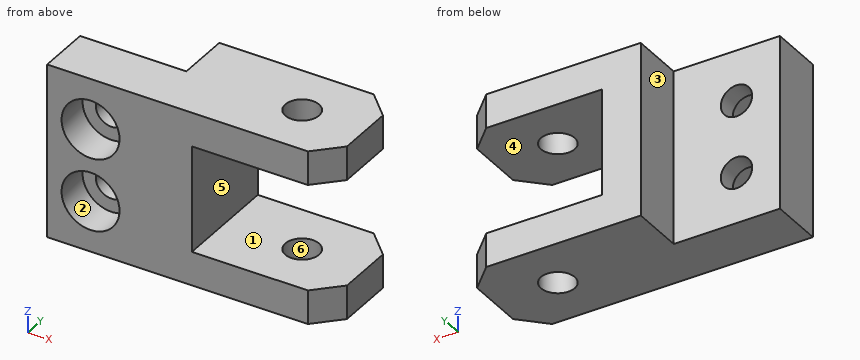
```python
from build123d import *

# Parameters (mm, degrees)
ESQUISSE1_R                                     = 3.5
BASE_EXTRUSION_DEPTH                            = 36
CHAMBRAGE_POUR_VIS_T_TE_CYLINDRIQUE_D           = 6.5
CHAMBRAGE_POUR_VIS_T_TE_CYLINDRIQUE_CBORE_D     = 12
CHAMBRAGE_POUR_VIS_T_TE_CYLINDRIQUE_CBORE_DEPTH = 7
ENL_V_MAT_EXTRU_1_DEPTH                         = 29


with BuildPart() as part:
    # Esquisse1 → Base-Extrusion (new body)
    with BuildSketch(Plane.XY):
        Polygon((0, 0), (0, 11), (32, 11), (37, 6), (37, -6), (32, -11), (-22, -11), (-22, 0), align=None)
        with Locations((24, 0)):
            Circle(ESQUISSE1_R, mode=Mode.SUBTRACT)
    extrude(amount=-BASE_EXTRUSION_DEPTH)

    # Chambrage pour vis à tête cylindrique à 6 pans creux (vis CHC) M51 (through all)
    with Locations(Plane.XZ.offset(11)):
        with Locations((-13, -25.5), (-13, -10.5)):
            CounterBoreHole(CHAMBRAGE_POUR_VIS_T_TE_CYLINDRIQUE_D / 2, CHAMBRAGE_POUR_VIS_T_TE_CYLINDRIQUE_CBORE_D / 2, CHAMBRAGE_POUR_VIS_T_TE_CYLINDRIQUE_CBORE_DEPTH)

    # Esquisse4 → Enlèv. mat.-Extru.1 (cut)
    with BuildSketch(Plane(origin=(37, 0, 0), x_dir=(0, 0, -1), z_dir=(1, 0, 0))):
        Polygon((29, -12.973294334), (18, -12.973294334), (7, -12.973294334), (7, 12.026705666), (18, 12.026705666), (29, 12.026705666), align=None)
    extrude(amount=-ENL_V_MAT_EXTRU_1_DEPTH, mode=Mode.SUBTRACT)


solid = part.part
```
CAD build for the part. Positions are in the model's coordinates, mm. Face numbers are marked on the shaded views. A direction names the side the tool comes from. Round coordinates to 2 decimals unless told otherwise and drop trailing zeros. Order: outer loops, then holes, each group sorted by start corner. A loop starts at its lowest first (then second) coordinate and runs counter-clockwise, first axis right, second up. Notation, with made-up numbers: (31, 63.5) - (71, 63.5) arc R18 cw to (71, 76.5) - close; hole circle Ø11 at (65, -3.75). An arc over 180 degrees is marked (long way). Use CSV: the item, a comma, the result in double quotes. Start each with the question number.
1) Two-plate mould, pull along X, no slides. Class the marked faces 4, 5 and 6: pulls with the +X half, pulls with the -X half, needs draft (parallel to the pull), parting line crosses it, or undercut.
2) Wall check: L1, parallel to Z at x = -13, y = -7.25; L2, parallel to Z at x = 10, y = -10; L3, parallel to Z at x = -13, y = -2.85. Give the ranges that are in metal, low to high. Write a range as [from, to].
3) Tool access for the marked faces 1, 2 and 3: list every direction of +Z, -Z, +X, -X, +Y, -Y with a clear straight run to the whole face (end or side of a thin tool).
4) Pin check, flat tips, straight feed: pin 1 Ø6 at (x, y) = (19.5, 5) entering from +Z; pin 2 Ø8.5 at (x, z) = (-13, -10.5) entering from +Y; pin 3 Ø6 at (y, z) = (7.5, -24) entering from -X; pin 4 Ø11 at (y, z) = (0.5, -13) entering from +X. Stop position of each tip, or through.
5) Saw through at D-D (y = 2.75). List the corners of the cut face in (x, z), and give its area (3 significant figures).
6) Saw through at B-B (z = -2.5). List the corners of the cut face in (x, y).
7) Saw through at A-A (x = 12). List the corners of the cut face in (y, z).
8) Saw through at C-C (x = -13). List the corners of the cut face in (y, z), and give its area (3 significant figures).
Values follow:
1,face 4,"needs draft"
1,face 5,"pulls with the +X half"
1,face 6,"undercut"
2,L1,"z = [-36, -31.5], [-19.5, -16.5], [-4.5, 0]"
2,L2,"z = [-36, -29], [-7, 0]"
2,L3,"z = [-36, -28.75], [-22.25, -13.75], [-7.25, 0]"
3,face 1,"+X, +Y, -Y"
3,face 2,"-Y"
3,face 3,"+Z, -Z, -X, +Y"
4,pin 1,"stops at z = 0"
4,pin 2,"stops at y = 0"
4,pin 3,"stops at x = 0"
4,pin 4,"stops at x = 8"
5,outline,"(0, -36) - (21.83, -36) - (21.83, -29) - (8, -29) - (8, -7) - (21.83, -7) - (21.83, 0) - (0, 0) - close; (26.17, -36) - (37, -36) - (37, -29) - (26.17, -29) - close; (26.17, -7) - (37, -7) - (37, 0) - (26.17, 0) - close"
5,area,"633 mm2"
6,outline,"(-22, -11) - (32, -11) - (37, -6) - (37, 6) - (32, 11) - (0, 11) - (0, 0) - (-22, 0) - close; hole circle Ø7 at (24, 0)"
7,outline,"(-11, -36) - (11, -36) - (11, -29) - (-11, -29) - close; (-11, -7) - (11, -7) - (11, 0) - (-11, 0) - close"
8,outline,"(-11, -36) - (0, -36) - (0, -28.75) - (-4, -28.75) - (-4, -31.5) - (-11, -31.5) - close; (-11, -19.5) - (-4, -19.5) - (-4, -22.25) - (0, -22.25) - (0, -13.75) - (-4, -13.75) - (-4, -16.5) - (-11, -16.5) - close; (-11, -4.5) - (-4, -4.5) - (-4, -7.25) - (0, -7.25) - (0, 0) - (-11, 0) - close"
8,area,"176 mm2"
